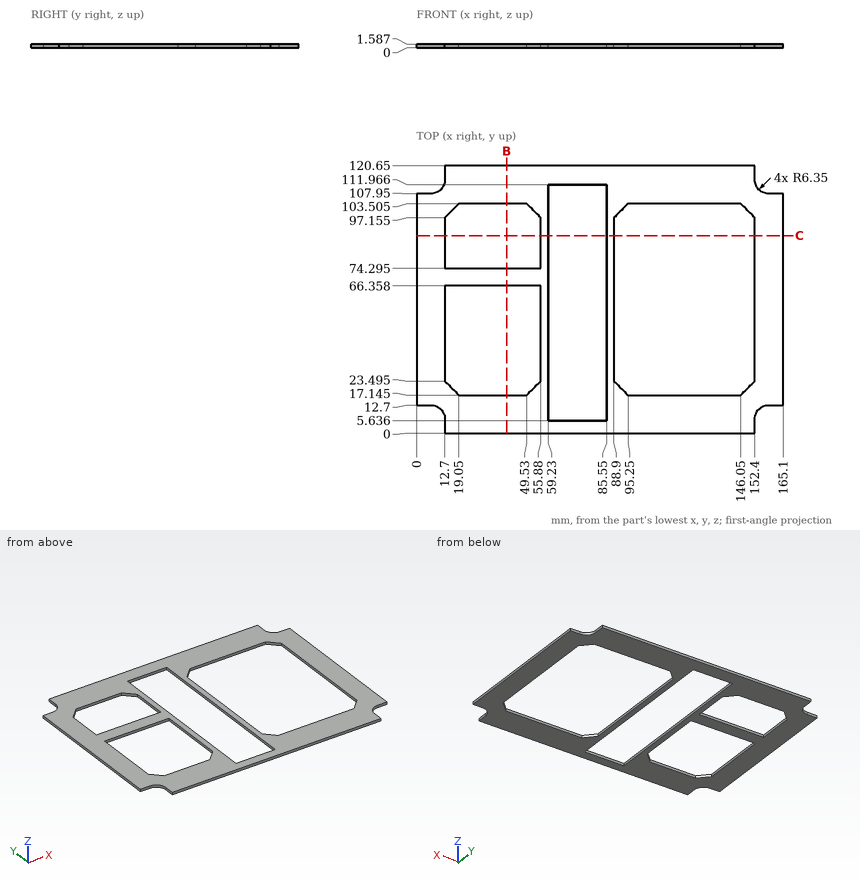
Source: three-view drawing plus pictorial views. Frame: mm from the lowest corner of the part. Coordinates: 2 decimals unless noted, no trailing zeros. Write each loop counter-clockwise with the first axis right and the second up, starting at its lowest first coordinate (ties: lowest second). Pieces come first, ordered by that corner, then holes. Notation, with made-up numbers: (1, 61.25) -> (25, 61.25) arc R13 ccw to (25, 86.25) -> close; hole circle Ø10 at (37, -10). An arc over 180 degrees is marked (long way). Write each question's results on one line, items separated by ' | '.
Item 1: Material intervals for probe 1 along X at (y, z) = (38, 0.5); probe 2 along X at (y, z) = (14, 1.2); probe 3 along Y at (x, z) = (158.5, 1.2) (1 decimal), sorted ascending.
Conclusion:
probe 1: x = 0 to 12.7, 55.88 to 59.23, 85.55 to 88.9, 152.4 to 165.1 | probe 2: x = 0 to 59.23, 85.55 to 165.1 | probe 3: y = 12.7 to 108
Item 2: Section query C-C on y = 89. Return loops of the section in (x, z).
Conclusion:
outline: (0, 0) -> (12.7, 0) -> (12.7, 1.59) -> (0, 1.59) -> close; (55.88, 0) -> (59.23, 0) -> (59.23, 1.59) -> (55.88, 1.59) -> close; (85.55, 0) -> (88.9, 0) -> (88.9, 1.59) -> (85.55, 1.59) -> close; (152.4, 0) -> (165.1, 0) -> (165.1, 1.59) -> (152.4, 1.59) -> close
Item 3: Section query B-B on x = 40.5. Count the separate pieces of the cut face and the enclosed holes in it.
Conclusion:
separate pieces: 3 | enclosed holes: 0
Item 4: Pin query (flat end, axial travel): pin 1 Ø0.5 at (y, z) = (2, 1) entering from +X; pin 2 Ø0.5 at (x, z) = (161.5, 0.5) entering from -Y; pin 3 Ø12 at (x, y) = (66, 43) entering from -Z. Return the tip coordinate at first contact, or that it passes through.
Conclusion:
pin 1: stops at x = 152.4 | pin 2: stops at y = 12.7 | pin 3: passes through
